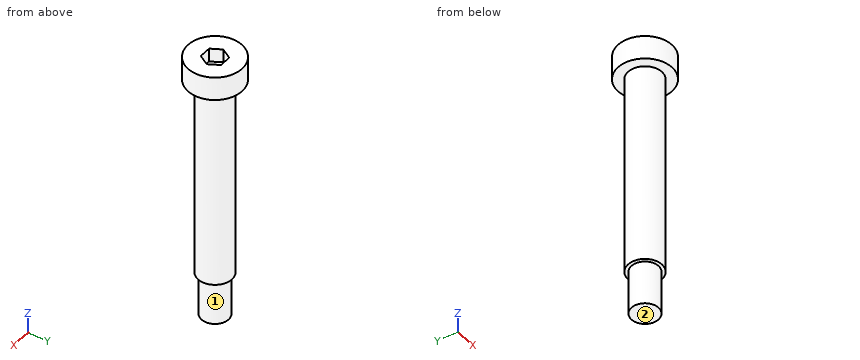
```python
from build123d import *

# Parameters (mm, degrees)
SKETCH1_R      = 2
THREAD_DEPTH   = 6.5
SKETCH2_R      = 2.5
SHOULDER_DEPTH = 30
SKETCH3_R      = 4
HEAD_DEPTH     = 3.5
SOCKET_DEPTH   = 2


with BuildPart() as part:
    # Sketch1 → Thread (new body)
    with BuildSketch(Plane.XY):
        Circle(SKETCH1_R)
    extrude(amount=THREAD_DEPTH)

    # Sketch2 → Shoulder (add)
    with BuildSketch(Plane.XY.offset(6.5)):
        Circle(SKETCH2_R)
    extrude(amount=SHOULDER_DEPTH)

    # Sketch3 → Head (add)
    with BuildSketch(Plane.XY.offset(36.5)):
        Circle(SKETCH3_R)
    extrude(amount=HEAD_DEPTH)

    # Sketch4 → Socket (cut)
    with BuildSketch(Plane.XY.offset(38)):
        Polygon((1.732050808, 0), (0.866025404, 1.5), (-0.866025404, 1.5), (-1.732050808, 0), (-0.866025404, -1.5), (0.866025404, -1.5), align=None)
    extrude(amount=SOCKET_DEPTH, mode=Mode.SUBTRACT)


solid = part.part
```
CAD build for the part. Positions are in the model's coordinates, mm. Face numbers are marked on the shaded views. A direction names the side the tool comes from. Round coordinates to 2 decimals unless told otherwise and drop trailing zeros. Order: outer loops, then holes, each group sorted by start corner. A loop starts at its lowest first (then second) coordinate and runs counter-clockwise, first axis right, second up.
Item 1: Pin check, flat tips, straight feed: pin 1 (2 mm diameter, centred on y = 3, z = 28, fed in from -X); pin 2 (3 mm diameter, centred on y = 3, z = 20.5, fed in from -X). Stop position of each tip, or through.
Item 2: Saw through at C-C on z = 10. Write the cut outline in (x, y), then the cut area to 3 significant figures.
Item 3: Probe line 1 along X through (y, z) = (1.5, 8); line 2 along Z through (x, y) = (3, -1). List the from-to ranges inside material, lowest first.
Item 4: Saw through at A-A on x = 0. Write the cut outline in (y, z), then the cut area to 3 significant figures.
Item 5: Tool access for the marked faces 1 and 2: list every direction of +Z, -Z, +X, -X, +Y, -Y with a clear straight run to the whole face (end or side of a thin tool).
Item 6: Saw through at B-B on y = 0.5. Write the cut outline in (x, z), then the cut area to 3 significant figures.
Item 7: Saw through at D-D on z = 5. Write the cut outline in (x, y), then the cut area to 3 significant figures.
Reported:
1. pin 1: stops at x = -1.5
1. pin 2: stops at x = -2
2. outline: circle Ø5 at (0, 0)
2. area: 19.6 mm2
3. line 1: x = -2 to 2
3. line 2: z = 36.5 to 40
4. outline: (-4, 36.5) - (-2.5, 36.5) - (-2.5, 6.5) - (-2, 6.5) - (-2, 0) - (2, 0) - (2, 6.5) - (2.5, 6.5) - (2.5, 36.5) - (4, 36.5) - (4, 40) - (1.5, 40) - (1.5, 38) - (-1.5, 38) - (-1.5, 40) - (-4, 40) - close
4. area: 198 mm2
5. face 1: -Z
5. face 2: -Z, +X, -X, +Y, -Y
6. outline: (-3.97, 36.5) - (-2.45, 36.5) - (-2.45, 6.5) - (-1.94, 6.5) - (-1.94, 0) - (1.94, 0) - (1.94, 6.5) - (2.45, 6.5) - (2.45, 36.5) - (3.97, 36.5) - (3.97, 40) - (1.44, 40) - (1.44, 38) - (-1.44, 38) - (-1.44, 40) - (-3.97, 40) - close
6. area: 194 mm2
7. outline: circle Ø4 at (0, 0)
7. area: 12.6 mm2
